For this review, take the finished solid that the model builds, in its own axes (mm). A direction names the side the tool comes from. Give positions to 0.01 mm unless a question says otherwise; leave off trailing zeros. Loops run counter-clockwise (first coordinate to the right, second up) from the corner with the lowest first, then second, coordinate; pieces in that order, holes last. Notation, with made-up numbers: (-38.5, 88) - (-10.5, 88) arc R17 cw to (-10.5, 108) - close; hole circle Ø10 at (61, 57). An arc over 180 degrees is marked (long way). Put each result on its own line as item: value.
from build123d import *

# Parameters (mm, degrees)
SKETCH1_R           = 44.45
SKETCH1_R_2         = 1.7
BOSS_EXTRUDE1_DEPTH = 2.794
SKETCH3_W           = 12.7
SKETCH3_H           = 5.08
BOSS_EXTRUDE2_DEPTH = 8.89
SKETCH4_R           = 1.778
CUT_EXTRUDE1_DEPTH  = 13.208
CIRPATTERN1_COUNT   = 2


with BuildPart() as part:
    # Sketch1 → Boss-Extrude1 (new body)
    with BuildSketch(Plane(origin=(0, 0, 0), x_dir=(1, 0, 0), z_dir=(0, 1, 0))):
        with Locations(Location((44.45, 44.45, 0), (0, 0, 270))):
            Circle(SKETCH1_R)
        with Locations(Location((65.31404504, 23.58595496, 0), (0, 0, 270))):
            Circle(SKETCH1_R_2, mode=Mode.SUBTRACT)
        with Locations(Location((23.58595496, 65.31404504, 0), (0, 0, 270))):
            Circle(SKETCH1_R_2, mode=Mode.SUBTRACT)
    extrude(amount=BOSS_EXTRUDE1_DEPTH)

    # Sketch3 → Boss-Extrude2 (add)
    with BuildSketch(Plane(origin=(0, 2.794, 0), x_dir=(1, 0, 0), z_dir=(0, 1, 0))):
        with Locations((44.99404504, 77.47)):
            Rectangle(SKETCH3_W, SKETCH3_H)
        with Locations((43.90595496, 11.43)):
            Rectangle(SKETCH3_W, SKETCH3_H)
    extrude(amount=BOSS_EXTRUDE2_DEPTH)

    # Sketch4 → Cut-Extrude1 (cut)
    with BuildSketch(Plane.XY.offset(-8.89)):
        with Locations((43.90595496, 7.366)):
            Circle(SKETCH4_R)
    cut_extrude1 = extrude(amount=-CUT_EXTRUDE1_DEPTH, mode=Mode.SUBTRACT)

    # CirPattern1: Cut-Extrude1 ×2 about axis
    cirpattern1_axis = Axis((44.45, 2.794, -44.45), (0, 1, 0))
    for i in range(1, CIRPATTERN1_COUNT):
        add(cut_extrude1.rotate(cirpattern1_axis, i * 360 / CIRPATTERN1_COUNT), mode=Mode.SUBTRACT)


solid = part.part
1) Take a section at D-D on z = -44.45. State the section outline as (x, y) points, and give its area (3 significant figures).
Geometry check:
outline: (0, 0) - (88.9, 0) - (88.9, 2.79) - (0, 2.79) - close
area: 248 mm²
2) Draft analysis for pull direction X (two halves, no side actions). For faces 1 (the face through (50.256, 7, -11)), 2 (the face through (42.13, 7.44, -11.39)), 3 (the face through (45, 0, -45)), state which applies: pulls with the +X half, pulls with the -X half, needs draft (parallel to the pull), parting line crosses it, or undercut.
Geometry check:
face 1: pulls with the +X half
face 2: undercut
face 3: needs draft
3) Take a section at B-B on x = 44.45. State the section outline as (y, z) points.
Geometry check:
outline: (0, -88.9) - (2.79, -88.9) - (2.79, -80.01) - (5.67, -80.01) - (5.67, -74.93) - (2.79, -74.93) - (2.79, -13.97) - (5.67, -13.97) - (5.67, -8.89) - (2.79, -8.89) - (2.79, 0) - (0, 0) - close; (9.06, -80.01) - (11.68, -80.01) - (11.68, -74.93) - (9.06, -74.93) - close; (9.06, -13.97) - (11.68, -13.97) - (11.68, -8.89) - (9.06, -8.89) - close
4) Wall thickness on line 1 (Y direction, x = 58, z = -57.5); line 2 (Z direction, x = 50, y = 3.75); line 3 (X direction, y = 6.75, z = -12.5): over which ranges is each line inside the solid? List them lowest first.
Geometry check:
line 1: y = 0 to 2.79
line 2: z = -80.01 to -74.93, -13.97 to -8.89
line 3: x = 37.56 to 42.24, 45.57 to 50.26
5) Take a section at C-C on z = -77. State the section outline as (x, y) points.
Geometry check:
outline: (14.18, 0) - (74.72, 0) - (74.72, 2.79) - (51.34, 2.79) - (51.34, 11.68) - (38.64, 11.68) - (38.64, 2.79) - (14.18, 2.79) - close; hole circle Ø3.56 at (44.99, 7.37)
6) Take a section at A-A on y = 10.25. State the section outline as (x, z) points, and give its area (3 significant figures).
Geometry check:
outline: (37.56, -13.97) - (50.26, -13.97) - (50.26, -8.89) - (37.56, -8.89) - close; (38.64, -80.01) - (51.34, -80.01) - (51.34, -74.93) - (38.64, -74.93) - close
area: 129 mm²
7) Insertion check: pin 1 Ø5.5 at (x, y) = (44.99, 7.37) entering from +Z; pin 2 Ø4.5 at (x, y) = (43, 9) entering from -Z; pin 3 Ø5.5 at (y, z) = (8.5, -76.5) entering from -X. Each pin has a flat end and moves straight along its axis. Give the tip position at first contact, or say it passes through.
Geometry check:
pin 1: stops at z = -8.89
pin 2: stops at z = -80.01
pin 3: stops at x = 38.64
8) For faces 4 (the face through (42, 6, -13.97)), 5 (the face through (38.644, 7, -77)), 6 (the face through (42, 6, -8.89)), 7 (the face through (43.35, 6.69, -77.51)), list the 3-axis set-ups (+Z, -Z, +X, -X, +Y, -Y) from which the entire face can be reached by the end or side of a thin tool; tool diameter is ignored.
Geometry check:
face 4: +X, -X, +Y
face 5: -Z, -X, +Y
face 6: +Z, +X, -X, +Y
face 7: -Z
